from build123d import *

# Parameters (mm, degrees)
SKETCH3_R           = 2.75
BOSS_EXTRUDE1_DEPTH = 3.175


with BuildPart() as part:
    # Sketch3 → Boss-Extrude1 (new body)
    with BuildSketch(Plane.XY):
        with BuildLine():
            Line((-151.387366014, 162.94696479), (-171.218095931, 153.699743563))
            ThreePointArc((-171.218095931, 153.699743563), (-178.553147236, 147.851921545), (-187.747718893, 145.99185379))
            Line((-187.747718893, 145.99185379), (-224.213491791, 128.987584627))
            Line((-224.213491791, 128.987584627), (-222.816572263, 123.774209976))
            Line((-222.816572263, 123.774209976), (-190.317469649, 123.774209976))
            Line((-190.317469649, 123.774209976), (-143.336488128, 145.681801447))
            Line((-143.336488128, 145.681801447), (-151.387366014, 162.94696479))
        make_face()
        with Locations((-157.41934736, 152.220574699)):
            Circle(SKETCH3_R, mode=Mode.SUBTRACT)
        with Locations((-203.641044499, 130.66704335)):
            Circle(SKETCH3_R, mode=Mode.SUBTRACT)
    extrude(amount=-BOSS_EXTRUDE1_DEPTH)


solid = part.part
Part model, mm, in its own coordinate system. Round coordinates to 2 decimals unless told otherwise and drop trailing zeros. Write each loop counter-clockwise with the first axis right and the second up, starting at its lowest first coordinate (ties: lowest second). Pieces come first, ordered by that corner, then holes. Notation, with made-up numbers: M 4,15 L 33,15 A19 cw 33,23 Z; hole C 56.25,48 d10. An arc over 180 degrees is marked long. Return JSON: item names as keys, results as strings. Group by question number.
(1) Saw through at D-D on y = 141.5. Write the cut outline in (x, z) (3 decimals), then the cut area to 3 significant figures.
(2) Pin check, flat tips, straight feed: pin 1 Ø12 at (x, y) = (-194.5, 151) entering from -Z; pin 2 Ø1.5 at (y, z) = (131, -2.5) entering from -X. Stop position of each tip, or through.
(3) Drill centre lines: probe 1 along X at (y, z) = (153, -2.05); probe 2 along X at (y, z) = (130.5, -0.7); probe 3 along X at (y, z) = (136.5, -1.7). Where is each one in solid material? Low to high.
(4) Saw through at A-A on y = 132. Write the cut outline in (x, z) (3 decimals), then the cut area to 3 significant figures.
(5) Saw through at C-C on z = -2.5. Write the cut outline in (x, y), then the cut area to 3 significant figures.
(6) Saw through at B-B on x = -158. Write the cut outline in (y, z) (3 decimals), then the cut area to 3 significant figures.
Returned:
{
 "1": {"outline": "M -197.381,-3.175 L -152.304,-3.175 L -152.304,0 L -197.381,0 Z", "area": "143 mm²"},
 "2": {"pin 1": "through", "pin 2": "x = -221.51"},
 "3": {"probe 1": "-171.79 to -160.06, -154.78 to -146.75", "probe 2": "-220.97 to -206.39, -200.9 to -175.89", "probe 3": "-208.1 to -163.03"},
 "4": {"outline": "M -217.753,-3.175 L -206.046,-3.175 L -206.046,0 L -217.753,0 Z; M -201.236,-3.175 L -172.677,-3.175 L -172.677,0 L -201.236,0 Z", "area": "128 mm²"},
 "5": {"outline": "M -224.21,128.99 L -222.82,123.77 L -190.32,123.77 L -143.34,145.68 L -151.39,162.95 L -171.22,153.7 A20 cw -187.75,145.99 Z; hole C -203.64,130.67 d5.5; hole C -157.42,152.22 d5.5", "area": "1,270 mm²"},
 "6": {"outline": "M 138.844,-3.175 L 149.533,-3.175 L 149.533,0 L 138.844,0 Z; M 154.909,-3.175 L 159.863,-3.175 L 159.863,0 L 154.909,0 Z", "area": "49.7 mm²"}
}
